from build123d import *

# Parameters (mm, degrees)
F0_W     = 150
F0_H     = 2
F0_R     = 2.5
F0_R_2   = 2.05
F0_R_3   = 1.2
F0_W_2   = 385
F0_H_2   = 56
F0_W_3   = 235
F0_H_3   = 3
F1_DEPTH = 3
F2_W     = 60
F2_H     = 150
F2_H_2   = 60
F2_H_3   = 550
F3_DEPTH = 25
F4_R     = 1.2
F5_DEPTH = 25


with BuildPart() as f1:
    # F0 (on Top) → F1 (new body)
    with BuildSketch(Plane.XY):
        with Locations((117.5, -54)):
            Rectangle(F0_W, F0_H)
        Polygon((42.5, -53), (192.5, -53), (192.5, 53), (-192.5, 53), (-192.5, -53), align=None)
        with Locations((-177.5, -7)):
            Circle(F0_R, mode=Mode.SUBTRACT)
        with Locations((-172.5, 43.5)):
            Circle(F0_R_2, mode=Mode.SUBTRACT)
        with Locations((-157.5, 43.5)):
            Circle(F0_R_2, mode=Mode.SUBTRACT)
        with Locations((-77.5, 43.5)):
            Circle(F0_R_2, mode=Mode.SUBTRACT)
        with Locations((-62.5, 43.5)):
            Circle(F0_R_2, mode=Mode.SUBTRACT)
        with Locations((27.5, -7)):
            Circle(F0_R, mode=Mode.SUBTRACT)
        with Locations((62.5, -43.417)):
            Circle(F0_R_2, mode=Mode.SUBTRACT)
        with Locations((77.5, -43.417)):
            Circle(F0_R_2, mode=Mode.SUBTRACT)
        with Locations((62.5, 43.5)):
            Circle(F0_R_2, mode=Mode.SUBTRACT)
        with Locations((77.5, 43.5)):
            Circle(F0_R_2, mode=Mode.SUBTRACT)
        with Locations((157.5, -43.417)):
            Circle(F0_R_2, mode=Mode.SUBTRACT)
        with Locations((172.5, -43.417)):
            Circle(F0_R_2, mode=Mode.SUBTRACT)
        with Locations((162.5, -7)):
            Circle(F0_R, mode=Mode.SUBTRACT)
        with Locations((157.5, 43.5)):
            Circle(F0_R_2, mode=Mode.SUBTRACT)
        with Locations((172.5, 43.5)):
            Circle(F0_R_2, mode=Mode.SUBTRACT)
        Polygon((42.5, -55), (42.5, -53), (-192.5, -53), (-192.5, -559.6), (42.5, -559.6), align=None)
        with Locations((-172.5, -550.1)):
            Circle(F0_R_2, mode=Mode.SUBTRACT)
        with Locations((-157.5, -550.1)):
            Circle(F0_R_2, mode=Mode.SUBTRACT)
        with Locations((-177.5, -499.6)):
            Circle(F0_R, mode=Mode.SUBTRACT)
        with Locations((-134.5, -544.6)):
            Circle(F0_R, mode=Mode.SUBTRACT)
        with Locations((-77.5, -550.1)):
            Circle(F0_R_2, mode=Mode.SUBTRACT)
        with Locations((-62.5, -550.1)):
            Circle(F0_R_2, mode=Mode.SUBTRACT)
        with Locations((-17.5, -544.6)):
            Circle(F0_R, mode=Mode.SUBTRACT)
        with Locations((-172.5, -339.6)):
            Circle(F0_R_3, mode=Mode.SUBTRACT)
        with Locations((-62.5, -339.6)):
            Circle(F0_R_3, mode=Mode.SUBTRACT)
        with Locations((27.5, -499.6)):
            Circle(F0_R, mode=Mode.SUBTRACT)
        with Locations((-177.5, -199.6)):
            Circle(F0_R, mode=Mode.SUBTRACT)
        with Locations((-172.5, -167)):
            Circle(F0_R_3, mode=Mode.SUBTRACT)
        with Locations((-62.5, -167)):
            Circle(F0_R_3, mode=Mode.SUBTRACT)
        with Locations((27.5, -199.6)):
            Circle(F0_R, mode=Mode.SUBTRACT)
        with Locations((0, 81)):
            Rectangle(F0_W_2, F0_H_2)
        with Locations((-132.5, 78)):
            Circle(F0_R, mode=Mode.SUBTRACT)
        with Locations((-17.5, 78)):
            Circle(F0_R, mode=Mode.SUBTRACT)
        with Locations((132.5, 78)):
            Circle(F0_R, mode=Mode.SUBTRACT)
        with Locations((-75, -561.1)):
            Rectangle(F0_W_3, F0_H_3)
    extrude(amount=F1_DEPTH)

    # F2 (on face) → F3 (cut)
    with BuildSketch(Plane.XY.offset(3)):
        with Locations((-117.5, -47)):
            Rectangle(F2_W, F2_H)
        with Locations((-117.5, -247)):
            Rectangle(F2_W, F2_H)
        with Locations((117.5, 0)):
            Rectangle(F2_W, F2_H_2)
        with Locations((-117.5, -447)):
            Rectangle(F2_W, F2_H)
        with Locations((-17.5, -247)):
            Rectangle(F2_W, F2_H_3)
    extrude(amount=-F3_DEPTH, mode=Mode.SUBTRACT)

    # F4 (on face) → F5 (cut)
    with BuildSketch(Plane.XY.offset(3)):
        with Locations((-180.5, 94)):
            Circle(F4_R)
        with Locations((-180.5, 74)):
            Circle(F4_R)
        with Locations((-180.5, -446)):
            Circle(F4_R)
        with Locations((-180.5, -466)):
            Circle(F4_R)
        with Locations((30.5, -446)):
            Circle(F4_R)
        with Locations((30.5, -466)):
            Circle(F4_R)
        with Locations((30.5, -76)):
            Circle(F4_R)
        with Locations((30.5, -96)):
            Circle(F4_R)
        with Locations((180.5, 94)):
            Circle(F4_R)
        with Locations((180.5, 74)):
            Circle(F4_R)
        with Locations((180.5, 9)):
            Circle(F4_R)
        with Locations((180.5, -11)):
            Circle(F4_R)
        with Locations((-114.5, -552.1)):
            Circle(F4_R)
        with Locations((-94.5, -552.1)):
            Circle(F4_R)
        with Locations((5.5, -552.1)):
            Circle(F4_R)
        with Locations((25.5, -552.1)):
            Circle(F4_R)
        with Locations((-112.5, 97)):
            Circle(F4_R)
        with Locations((-92.5, 97)):
            Circle(F4_R)
        with Locations((92.5, 97)):
            Circle(F4_R)
        with Locations((112.5, 97)):
            Circle(F4_R)
        with Locations((107.5, -43.8)):
            Circle(F4_R)
        with Locations((127.5, -43.8)):
            Circle(F4_R)
    extrude(amount=-F5_DEPTH, mode=Mode.SUBTRACT)


solid = f1.part
The listing builds one solid part. Answer for the finished solid, in the listing's coordinates (mm). Give positions to 0.01 mm unless a question says otherwise; leave off trailing zeros. Loops run counter-clockwise (first coordinate to the right, second up) from the corner with the lowest first, then second, coordinate; pieces in that order, holes last.
Item 1: A cutting plane is placed at B-B (y = -283). Give the vertices of the cut face in (x, z), then the cut area to 3 significant figures.
Derived:
outline: (-192.5, 0) - (-147.5, 0) - (-147.5, 3) - (-192.5, 3) - close; (-87.5, 0) - (-47.5, 0) - (-47.5, 3) - (-87.5, 3) - close; (12.5, 0) - (42.5, 0) - (42.5, 3) - (12.5, 3) - close
area: 345 mm2
Item 2: A cutting plane is placed at A-A (y = -141.5). Give the vertices of the cut face in (x, z), then the cut area to 3 significant figures.
Derived:
outline: (-192.5, 0) - (-47.5, 0) - (-47.5, 3) - (-192.5, 3) - close; (12.5, 0) - (42.5, 0) - (42.5, 3) - (12.5, 3) - close
area: 525 mm2
Item 3: Find the intervals of material crossed by line 1 along X through (y, z) = (-466, 1.4); line 2 along Y through (x, z) = (-177.5, 0.85); line 3 along X through (y, z) = (-499.6, 2.3), in increasing order.
Derived:
line 1: x = -192.5 to -181.7, -179.3 to -147.5, -87.5 to -47.5, 12.5 to 29.3, 31.7 to 42.5
line 2: y = -562.6 to -502.1, -497.1 to -202.1, -197.1 to -9.5, -4.5 to 109
line 3: x = -192.5 to -180, -175 to -147.5, -87.5 to -47.5, 12.5 to 25, 30 to 42.5
Item 4: This flat-tipped pin is pushed along its axis until it touches: pin 1 Ø0.9 at (y, z) = (-163, 1) entering from +X. Where does it stop, or does it pass through?
Derived:
pin 1: stops at x = 42.5
Item 5: A cutting plane is placed at C-C (x = -5). Give the vertices of the cut face in (y, z), then the cut area to 3 significant figures.
Derived:
outline: (-562.6, 0) - (-522, 0) - (-522, 3) - (-562.6, 3) - close; (28, 0) - (109, 0) - (109, 3) - (28, 3) - close
area: 365 mm2
Item 6: A cutting plane is placed at D-D (z = 1.95). Give the number of separate pieces and of enclosed holes in the cut face, then the cut area to 3 significant figures.
Derived:
separate pieces: 1
enclosed holes: 59
area: 118,000 mm2
